For this review, take the finished solid that the model builds, in its own axes (mm). Face numbers are marked on the shaded views. A direction names the side the tool comes from. Give positions to 0.01 mm unless a question says otherwise; leave off trailing zeros. Order: outer loops, then holes, each group sorted by start corner. A loop starts at its lowest first (then second) coordinate and runs counter-clockwise, first axis right, second up. Notation, with made-up numbers: M 73.5,67 L 130.5,67 A19 cw 130.5,79 Z; hole C -24,32.25 d1. An arc over 180 degrees is marked long. Answer as CSV lines item,"result". Start each with the question number.
1. We need section C-C, the plane y = 30.5. Give the boundary of the cut face in (x, z), and give its area (3 significant figures).
2. For line 1 along X through (y, z) = (12.5, -32.5); line 2 along Z through (x, y) = (-80, 7.5); line 3 along X through (y, z) = (4, -49.5), list the stretches that pass through material, from the lowest coordinate up.
3. Mouldability with a two-part tool opening along X and no side actions: class the marked faces 5, 6 and 7 as pulls with the +X half, pulls with the -X half, needs draft (parallel to the pull), parting line crosses it, or undercut.
4. Clearance check with flat-ended pins moving along their axes: P1, Ø6.5, axis at x = -68, z = -19.5, coming from the +Y side; P2, Ø4.5, axis at y = 4.5, z = -7, coming from the -X side; P3, Ø0.7, axis at x = -35, y = 1.5, coming from the +Z side; P4, Ø2, axis at x = -101, y = 3.5, coming from the -Z side. State where each tip first meets the part, or that it passes through.
5. We need section D-D, the plane z = 23. State how many separate pieces and enclosed holes the cut face has, and give its area (3 significant figures).
6. We need section B-B, the plane x = 32.5. Give the boundary of the cut face in (y, z).
7. We need section A-A, the plane x = -99.5. Give the boundary of the cut face in (y, z), and give its area (3 significant figures).
8. Machinability: for the marked faces 1, 2, 3 and 4, which of the approach directions +Z, -Z, +X, -X, +Y, -Y give a long, thin tool a straight path to every point of the face, cutting with its end or side? Answer none if there is none.
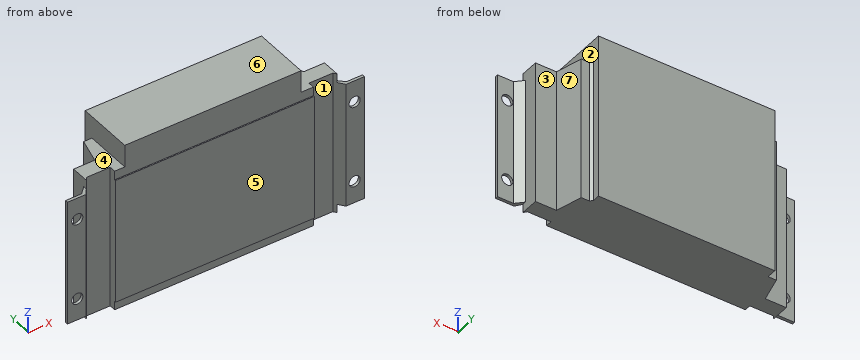
from build123d import *

# Parameters (mm, degrees)
SKETCH7_W           = 213
SKETCH7_H           = 90.5
BOSS_EXTRUDE1_DEPTH = 2
BOSS_EXTRUDE2_DEPTH = 40.9
CHAMFER1_SIZE       = 5
CUT_EXTRUDE1_DEPTH  = 166.359184807
CUT_EXTRUDE2_DEPTH  = 166.359184807
SKETCH11_R          = 4
CUT_EXTRUDE3_DEPTH  = 40.9


with BuildPart() as part:
    # Sketch7 → Boss-Extrude1 (new body)
    with BuildSketch(Plane(origin=(0, 0, 0), x_dir=(1, 0, 0), z_dir=(0, 1, 0))):
        with Locations((0, 8.157414363)):
            Rectangle(SKETCH7_W, SKETCH7_H)
    extrude(amount=BOSS_EXTRUDE1_DEPTH)

    # Sketch8 → Boss-Extrude2 (add)
    with BuildSketch(Plane(origin=(0, 2, 0), x_dir=(1, 0, 0), z_dir=(0, 1, 0))):
        Polygon((-90, 59.5), (-90, -43.5), (-64.043073189, -43.5), (-64.043073189, -59.5), (62.450636704, -59.5), (62.450636704, -43.5), (90, -43.5), (90, 59.5), align=None)
    extrude(amount=BOSS_EXTRUDE2_DEPTH)

    # Chamfer1
    chamfer1_edges = [part.edges().sort_by_distance(p)[0] for p in [
        (90, 2, -8.157414363),
        (-90, 2, -8.157414363),
    ]]
    chamfer(chamfer1_edges, length=CHAMFER1_SIZE)

    # Sketch9 → Cut-Extrude1 (cut, through all)
    with BuildSketch(Plane.XY.offset(59.5)):
        Polygon((-93.291667838, 0), (-88.36780993, 6.554671328), (-71.309248996, 6.554671328), (-71.309248996, 1.137273466), (71.309248996, 1.137273466), (71.309248996, 6.554671328), (88.36780993, 6.554671328), (93.291667838, 0), (93.291667838, -4.012269233), (-93.291667838, -4.012269233), align=None)
    extrude(amount=-CUT_EXTRUDE1_DEPTH, mode=Mode.SUBTRACT)

    # Sketch10 → Cut-Extrude2 (cut, through all)
    with BuildSketch(Plane.XY.offset(59.5)):
        Polygon((-90, 53.559109073), (-90, 17.435932261), (-74.881220668, 17.435932261), (-70.000468563, 35.913866357), (-64.043073189, 35.913866357), (-64.043073189, 42.9), (-58.569611619, 42.9), (58.569611619, 42.9), (62.450636704, 42.9), (62.450636704, 37.946396222), (64.043073189, 35.913866357), (70.000468563, 35.913866357), (74.881220668, 17.435932261), (90, 17.435932261), (90, 53.559109073), align=None)
    extrude(amount=-CUT_EXTRUDE2_DEPTH, mode=Mode.SUBTRACT)

    # Sketch11 → Cut-Extrude3 (cut)
    with BuildSketch(Plane(origin=(0, 2, 0), x_dir=(1, 0, 0), z_dir=(0, 1, 0))):
        with Locations(Location((99.5, 37.657414363, 0), (0, 0, 270))):
            Circle(SKETCH11_R)
        with Locations(Location((-99.5, 37.657414363, 0), (0, 0, 270))):
            Circle(SKETCH11_R)
        with Locations(Location((-99.5, -21.342585637, 0), (0, 0, 90))):
            Circle(SKETCH11_R)
        with Locations(Location((99.5, -21.342585637, 0), (0, 0, 90))):
            Circle(SKETCH11_R)
    extrude(amount=-CUT_EXTRUDE3_DEPTH, mode=Mode.SUBTRACT)


solid = part.part
Result set:
1,outline,"M -71.43,-59.5 L 71.43,-59.5 L 71.43,43.5 L 62.45,43.5 L 62.45,59.5 L -64.04,59.5 L -64.04,43.5 L -71.43,43.5 Z"
1,area,"16,700 mm2"
2,line 1,"-90 to 90"
2,line 2,"-59.5 to 43.5"
2,line 3,"-93 to -90.29, -71.31 to 71.31, 90.29 to 93"
3,face 5,"undercut"
3,face 6,"needs draft"
3,face 7,"pulls with the +X half"
4,P1,"y = 35.91"
4,P2,"x = -94.75"
4,P3,"z = 37.09"
4,P4,"through"
5,separate pieces,"3"
5,enclosed holes,"0"
5,area,"6,340 mm2"
6,outline,"M 1.14,-53.41 L 2,-53.41 L 2,-59.5 L 42.9,-59.5 L 42.9,59.5 L 2,59.5 L 2,37.09 L 1.14,37.09 Z"
7,outline,"M 0,-53.41 L 2,-53.41 L 2,-41.66 L 0,-41.66 Z; M 0,-33.66 L 2,-33.66 L 2,17.34 L 0,17.34 Z; M 0,25.34 L 2,25.34 L 2,37.09 L 0,37.09 Z"
7,area,"149 mm2"
8,face 1,"+Z, -Z, -Y"
8,face 2,"+Z, +X, +Y"
8,face 3,"+Z, -Z, +X, +Y"
8,face 4,"+Z, -X, +Y, -Y"
